```python
from build123d import *

# Parameters (mm, degrees)
F0_R     = 10
F0_R_2   = 6.5
F0_R_3   = 26
F0_R_4   = 5.5
F0_R_5   = 55
F0_R_6   = 11
F0_R_7   = 105
F0_R_8   = 2.5
F0_R_9   = 18.5
F0_R_10  = 3.75
F1_DEPTH = 25
F2_R     = 107.5
F3_DEPTH = 22
F4_R     = 162.5
F4_R_2   = 120
F5_DEPTH = 5


with BuildPart() as f1:
    # F0 (on Right) → F1 (new body)
    with BuildSketch(Plane.YZ):
        Polygon((255.000028, -215.000014), (255.000028, 189.999986), (230.000028, 214.999986), (-329.999972, 214.999986), (-354.999972, 189.999986), (-354.999972, -14.644675), (-347.677642, -32.322345), (-147.322303, -232.677684), (-129.644633, -240.000014), (230.000028, -240.000014), align=None)
        with Locations((-99.999965, -195.000014)):
            Circle(F0_R, mode=Mode.SUBTRACT)
        with BuildLine():
            ThreePointArc((-178.574351, -145), (-186.228019, -143.477591), (-192.716486, -139.142136))
            Line((-192.716486, -139.142136), (-272.546106, -59.312516))
            ThreePointArc((-272.546106, -59.312516), (-277.602171, -39.564214), (-262.713262, -25.640147))
            Line((-262.713262, -25.640147), (-164.601156, -3.991986))
            ThreePointArc((-164.601156, -3.991986), (-150.180759, -6.266335), (-141.147572, -17.734643))
            Line((-141.147572, -17.734643), (-131.216492, -50.584924))
            ThreePointArc((-131.216492, -50.584924), (-125.261921, -64.044001), (-116.21002, -75.648602))
            Line((-116.21002, -75.648602), (-81.000757, -110.857864))
            ThreePointArc((-81.000757, -110.857864), (-76.665302, -132.653669), (-95.142893, -145))
            Line((-95.142893, -145), (-178.574351, -145))
        make_face(mode=Mode.SUBTRACT)
        with Locations((225.000024, -210.000012)):
            Circle(F0_R_2, mode=Mode.SUBTRACT)
        with Locations((145.000028, -145.000014)):
            Circle(F0_R_3, mode=Mode.SUBTRACT)
        with Locations((-310.336309, 25.663677)):
            Circle(F0_R_4, mode=Mode.SUBTRACT)
        with Locations((-252, 1.499986)):
            Circle(F0_R_4, mode=Mode.SUBTRACT)
        with Locations((-334.5, 83.999986)):
            Circle(F0_R_4, mode=Mode.SUBTRACT)
        with Locations((-252, 83.999986)):
            Circle(F0_R_5, mode=Mode.SUBTRACT)
        with Locations((-193.663691, 25.663677)):
            Circle(F0_R_4, mode=Mode.SUBTRACT)
        with Locations((-169.5, 83.999986)):
            Circle(F0_R_4, mode=Mode.SUBTRACT)
        with Locations((-310.336309, 142.336296)):
            Circle(F0_R_4, mode=Mode.SUBTRACT)
        with Locations((-324.999969, 184.999984)):
            Circle(F0_R_2, mode=Mode.SUBTRACT)
        with Locations((-294.999969, 184.999984)):
            Circle(F0_R_6, mode=Mode.SUBTRACT)
        with Locations((-252, 166.499986)):
            Circle(F0_R_4, mode=Mode.SUBTRACT)
        with Locations((-193.663691, 142.336296)):
            Circle(F0_R_4, mode=Mode.SUBTRACT)
        Circle(F0_R_7, mode=Mode.SUBTRACT)
        with BuildLine():
            ThreePointArc((205, 82), (219.142136, 76.142136), (225, 62))
            Line((225, 62), (225, -63.360385))
            ThreePointArc((225, -63.360385), (214.713957, -80.842921), (194.436095, -80.342844))
            Line((194.436095, -80.342844), (154.436095, -55.460924))
            ThreePointArc((154.436095, -55.460924), (147.517464, -48.192421), (145, -38.478465))
            Line((145, -38.478465), (145, 62))
            ThreePointArc((145, 62), (150.857864, 76.142136), (165, 82))
            Line((165, 82), (205, 82))
        make_face(mode=Mode.SUBTRACT)
        with BuildLine():
            Line((-124.602032, 185), (68.436239, 185))
            ThreePointArc((68.436239, 185), (82.578374, 179.142136), (88.436239, 165))
            Line((88.436239, 165), (88.436239, 132.530642))
            ThreePointArc((88.436239, 132.530642), (79.651422, 115.971063), (61.014273, 113.95877))
            Line((61.014273, 113.95877), (31.989488, 125.558083))
            ThreePointArc((31.989488, 125.558083), (-0.279211, 132.581472), (-33.075883, 128.711678))
            Line((-33.075883, 128.711678), (-99.973507, 109.233479))
            ThreePointArc((-99.973507, 109.233479), (-113.421324, 110.043894), (-123.304149, 119.199785))
            Line((-123.304149, 119.199785), (-142.341565, 155.763715))
            ThreePointArc((-142.341565, 155.763715), (-141.700653, 175.374833), (-124.602032, 185))
        make_face(mode=Mode.SUBTRACT)
        with Locations((170.000028, 114.999986)):
            Circle(F0_R_8, mode=Mode.SUBTRACT)
        with Locations((184.547028, 104.131986)):
            Circle(F0_R_8, mode=Mode.SUBTRACT)
        with Locations((140.000028, 159.999986)):
            Circle(F0_R_9, mode=Mode.SUBTRACT)
        with Locations((170.000028, 159.999986)):
            Circle(F0_R_10, mode=Mode.SUBTRACT)
        with Locations((225.000024, 184.999984)):
            Circle(F0_R_2, mode=Mode.SUBTRACT)
    extrude(amount=F1_DEPTH)

    # F2 (on face) → F3 (cut)
    with BuildSketch(Plane.YZ.offset(25)):
        Circle(F2_R)
    extrude(amount=-F3_DEPTH, mode=Mode.SUBTRACT)

    # F4 (on face) → F5 (cut)
    with BuildSketch(Plane.YZ.offset(25)):
        Circle(F4_R)
        Circle(F4_R_2, mode=Mode.SUBTRACT)
    extrude(amount=-F5_DEPTH, mode=Mode.SUBTRACT)


solid = f1.part
```
Geometry: final body of the model. Coordinates: model frame, mm. A direction names the side the tool comes from. Coordinates: 2 decimals unless noted, no trailing zeros. Order: outer loops, then holes, each group sorted by start corner. A loop starts at its lowest first (then second) coordinate and runs counter-clockwise, first axis right, second up. Notation, with made-up numbers: (-37, 49.5) - (21, 49.5) arc R29 ccw to (21, 70.5) - close; hole circle Ø5 at (89.5, 19.25). An arc over 180 degrees is marked (long way). Return JSON: item names as keys, results as strings. Group by question number.
1. Cut plane A-A (y = 0). Output: boundary loops of the cut face in (x, z), plus the area to 3 significant figures.
2. Material intervals for line 1 along Y through (x, z) = (11.5, 183.5); line 2 along Y through (x, z) = (19, 91); line 3 along Z through (x, y) = (1.8, 0), sorted ascending. Write a range as [from, to].
3. Cut plane C-C (x = 9.25). Count the separate pieces of the cut face and the enclosed holes in it, plus the area to 3 significant figures.
4. Pull-direction query (Z, two-part tool) for faces 1 (the face through (12, 255, -15)), 2 (the face through (12, 242, -228)), 3 (the face through (12, -342, 203)), 4 (the face through (9.55, 147.59, -48.32)); classes: pulls with the +Z half, pulls with the -Z half, needs draft (parallel to the pull), parting line crosses it, or undercut.
5. Set-up query: faces 5 (the face through (12, 48, -240)), 6 (the face through (14.15, -85.31, -65.41)), 7 (the face through (9.86, 79.88, 116.13)). Return all of +Z, -Z, +X, -X, +Y, -Y with unobstructed straight access to the full face (end or side cutting, diameter ignored); none if empty.
6. Pin query (flat end, axial travel): pin 1 (11.5 mm diameter, centred on y = 225, z = 185, fed in from -X); pin 2 (1 mm diameter, centred on x = 10.5, z = -176, fed in from -Y). Return the tip coordinate at first contact, or that it passes through.
7. Cut plane B-B (z = -96). Output: boundary loops of the cut face in (x, y), plus the area to 3 significant figures.
Resolved:
{
 "1": {"outline": "(0, -240) - (25, -240) - (25, -162.5) - (20, -162.5) - (20, -120) - (25, -120) - (25, -107.5) - (3, -107.5) - (3, -105) - (0, -105) - close; (0, 105) - (3, 105) - (3, 107.5) - (25, 107.5) - (25, 120) - (20, 120) - (20, 132.57) - (0, 132.57) - close; (0, 185) - (25, 185) - (25, 215) - (0, 215) - close", "area": "4,430 mm²"},
 "2": {"line 1": "y = [-355, -331.32], [-318.68, -305.9], [-284.1, -132.2], [76.04, 218.68], [231.32, 255]", "line 2": "y = [-355, -306.55], [-197.45, -57.23], [57.23, 255]", "line 3": "z = [-240, -105], [105, 132.57], [185, 215]"},
 "3": {"separate pieces": "1", "enclosed holes": "23", "area": "158,000 mm²"},
 "4": {"face 1": "needs draft", "face 2": "pulls with the -Z half", "face 3": "pulls with the +Z half", "face 4": "undercut"},
 "5": {"face 5": "-Z, +X, -X, +Y, -Y", "face 6": "+X", "face 7": "+X, -X"},
 "6": {"pin 1": "passes through", "pin 2": "stops at y = -204.5"},
 "7": {"outline": "(0, -284) - (25, -284) - (25, -235.86) - (0, -235.86) - close; (0, -95.86) - (20, -95.86) - (20, -72) - (25, -72) - (25, -48.38) - (3, -48.38) - (3, -42.53) - (0, -42.53) - close; (0, 42.53) - (3, 42.53) - (3, 48.38) - (25, 48.38) - (25, 72) - (20, 72) - (20, 131.11) - (25, 131.11) - (25, 255) - (0, 255) - close", "area": "7,180 mm²"}
}
